```python
from build123d import *

# Parameters (mm, degrees)
V3_BOX_FOOTPRINT_100_X_45_MM_W                 = 100
V3_BOX_FOOTPRINT_100_X_45_MM_H                 = 45
V3_BOX_HEIGHT_35_MM_DEPTH                      = 35
V3_REAR_OPENING_96_X_31_MM_W                   = 96
V3_REAR_OPENING_96_X_31_MM_H                   = 31
V3_CAVITY_ALL_WALLS_2_MM_DEPTH                 = 43
V3_SQUARE_BEAMS_10_X_10_PITCH_95_MM_W          = 10
V3_SQUARE_BEAMS_10_X_10_PITCH_95_MM_H          = 10
V3_FORWARD_BEAM_LENGTH_65_MM_DEPTH             = 65
V3_LEFT_PCB_EAR_PROFILE_W                      = 10
V3_LEFT_PCB_EAR_PROFILE_H                      = 10
V3_LEFT_INWARD_EAR_5_MM_DEPTH                  = 5
V3_RIGHT_PCB_EAR_PROFILE_W                     = 10
V3_RIGHT_PCB_EAR_PROFILE_H                     = 10
V3_RIGHT_INWARD_EAR_5_MM_DEPTH                 = 5
V3_PCB_ROOF_PAIR_PITCH_85_MM_R                 = 1.7
V3_M3_ROOF_HOLES_DIAMETER_3_4_MM_DEPTH         = 2
V3_PCB_FORWARD_PAIR_ROW_SPACING_60_MM_R        = 1.7
V3_M3_PCB_EAR_HOLES_DEPTH                      = 10
V3_CHASSIS_TOP_HOLES_WIDTH_95_DEPTH_40_M_R     = 1.7
V3_M3_BEAM_TOP_BOTTOM_HOLES_DEPTH              = 10
V3_HANGING_PLATE_OFFSET_26_THICKNESS_2_5_W     = 110
V3_HANGING_PLATE_OFFSET_26_THICKNESS_2_5_H     = 2.5
V3_MOUNTING_PLATE_DOWNWARD_15_MM_WIDTH_1_DEPTH = 15
FOUR_HORIZONTAL_SLOTS_3_4_X_5_4_MM_DEPTH       = 2.5
CUT_EXTRUDE_1_DEPTH                            = 93.059763198
H_CROSSMEMBER_10_X_10_MM_AT_BEAM_MIDPOIN_W     = 10
H_CROSSMEMBER_10_X_10_MM_AT_BEAM_MIDPOIN_H     = 10
H_CROSSMEMBER_85_MM_DEPTH                      = 85
LONGITUDINAL_START                             = -2
BEAM_CAVITIES_6_MM_WIDE_PRESERVING_SCREW_W     = 6
BEAM_CAVITIES_6_MM_WIDE_PRESERVING_SCREW_H     = 6
BEAM_CAVITIES_6_MM_WIDE_PRESERVING_SCREW_H_2   = 27
BEAM_CAVITIES_6_MM_WIDE_PRESERVING_SCREW_H_3   = 9
LONGITUDINAL_BEAM_WALLS_2_MM_INNER_HEI_DEPTH   = 6
H_START                                        = -2
H_CROSSMEMBER_CAVITY_CONNECTS_BOTH_BEAM_W      = 89
H_CROSSMEMBER_CAVITY_CONNECTS_BOTH_BEAM_H      = 6
H_CROSSMEMBER_WALLS_2_MM_DEPTH                 = 6
CUT_EXTRUDE_4_DEPTH                            = 93.059763198
V6_EXTEND_10_X_10_HOLLOW_BEAMS_WITH_2_MM_W     = 10
V6_EXTEND_10_X_10_HOLLOW_BEAMS_WITH_2_MM_H     = 10
V6_EXTEND_10_X_10_HOLLOW_BEAMS_WITH_2_MM_W_2   = 6
V6_EXTEND_10_X_10_HOLLOW_BEAMS_WITH_2_MM_H_2   = 6
V6_HOLLOW_BEAM_EXTENSIONS_15_MM_DEPTH          = 15
V6_FOUR_FULL_DEPTH_PCB_PADS_CENTERS_X42_W      = 15
V6_FOUR_FULL_DEPTH_PCB_PADS_CENTERS_X42_H      = 10
V6_SOLID_SCREW_PADS_WITH_5_MM_INWARD_EAR_DEPTH = 10
V6_PCB_HOLES_85_X_60_MM_AND_RETAINED_CHA_R     = 1.7
V6_FOUR_PCB_M3_HOLES_THROUGH_REINFORCED_DEPTH  = 10


with BuildPart() as part:
    # V3 box footprint 100 x 45 mm → V3 box height 35 mm (new body)
    with BuildSketch(Plane.XY):
        with Locations((0, 22.5)):
            Rectangle(V3_BOX_FOOTPRINT_100_X_45_MM_W, V3_BOX_FOOTPRINT_100_X_45_MM_H)
    extrude(amount=V3_BOX_HEIGHT_35_MM_DEPTH)

    # V3 rear opening 96 x 31 mm → V3 cavity all walls 2 mm (cut)
    with BuildSketch(Plane(origin=(0, 45, 0), x_dir=(1, 0, 0), z_dir=(0, 1, 0))):
        with Locations((0, -17.5)):
            Rectangle(V3_REAR_OPENING_96_X_31_MM_W, V3_REAR_OPENING_96_X_31_MM_H)
    extrude(amount=-V3_CAVITY_ALL_WALLS_2_MM_DEPTH, mode=Mode.SUBTRACT)

    # V3 square beams 10 x 10 pitch 95 mm → V3 forward beam length 65 mm (add)
    with BuildSketch(Plane.XZ):
        with Locations((-47.5, 30)):
            Rectangle(V3_SQUARE_BEAMS_10_X_10_PITCH_95_MM_W, V3_SQUARE_BEAMS_10_X_10_PITCH_95_MM_H)
        with Locations((47.5, 30)):
            Rectangle(V3_SQUARE_BEAMS_10_X_10_PITCH_95_MM_W, V3_SQUARE_BEAMS_10_X_10_PITCH_95_MM_H)
    extrude(amount=V3_FORWARD_BEAM_LENGTH_65_MM_DEPTH)

    # V3 left PCB ear profile → V3 left inward ear 5 mm (add)
    with BuildSketch(Plane(origin=(-42.5, 0, 0), x_dir=(0, 0, -1), z_dir=(1, 0, 0))):
        with Locations((-30, -20)):
            Rectangle(V3_LEFT_PCB_EAR_PROFILE_W, V3_LEFT_PCB_EAR_PROFILE_H)
    extrude(amount=V3_LEFT_INWARD_EAR_5_MM_DEPTH)

    # V3 right PCB ear profile → V3 right inward ear 5 mm (add)
    with BuildSketch(Plane.ZY.offset(-42.5)):
        with Locations((30, -20)):
            Rectangle(V3_RIGHT_PCB_EAR_PROFILE_W, V3_RIGHT_PCB_EAR_PROFILE_H)
    extrude(amount=V3_RIGHT_INWARD_EAR_5_MM_DEPTH)

    # V3 PCB roof pair pitch 85 mm → V3 M3 roof holes diameter 3.4 mm (cut)
    with BuildSketch(Plane.XY.offset(35)):
        with Locations((-42.5, 40)):
            Circle(V3_PCB_ROOF_PAIR_PITCH_85_MM_R)
        with Locations((42.5, 40)):
            Circle(V3_PCB_ROOF_PAIR_PITCH_85_MM_R)
    extrude(amount=-V3_M3_ROOF_HOLES_DIAMETER_3_4_MM_DEPTH, mode=Mode.SUBTRACT)

    # V3 PCB forward pair row spacing 60 mm → V3 M3 PCB ear holes (cut)
    with BuildSketch(Plane.XY.offset(35)):
        with Locations((-42.5, -20)):
            Circle(V3_PCB_FORWARD_PAIR_ROW_SPACING_60_MM_R)
        with Locations((42.5, -20)):
            Circle(V3_PCB_FORWARD_PAIR_ROW_SPACING_60_MM_R)
    extrude(amount=-V3_M3_PCB_EAR_HOLES_DEPTH, mode=Mode.SUBTRACT)

    # V3 chassis top holes width 95 depth 40 mm → V3 M3 beam top bottom holes (cut)
    with BuildSketch(Plane.XY.offset(35)):
        with Locations((-47.5, -55)):
            Circle(V3_CHASSIS_TOP_HOLES_WIDTH_95_DEPTH_40_M_R)
        with Locations((-47.5, -15)):
            Circle(V3_CHASSIS_TOP_HOLES_WIDTH_95_DEPTH_40_M_R)
        with Locations((47.5, -55)):
            Circle(V3_CHASSIS_TOP_HOLES_WIDTH_95_DEPTH_40_M_R)
        with Locations((47.5, -15)):
            Circle(V3_CHASSIS_TOP_HOLES_WIDTH_95_DEPTH_40_M_R)
    extrude(amount=-V3_M3_BEAM_TOP_BOTTOM_HOLES_DEPTH, mode=Mode.SUBTRACT)

    # V3 hanging plate offset 26 thickness 2.5 mm → V3 mounting plate downward 15 mm width 110 (add)
    with BuildSketch(Plane(origin=(0, 0, 25), x_dir=(-1, 0, 0), z_dir=(0, 0, -1))):
        with Locations((0, -27.25)):
            Rectangle(V3_HANGING_PLATE_OFFSET_26_THICKNESS_2_5_W, V3_HANGING_PLATE_OFFSET_26_THICKNESS_2_5_H)
    extrude(amount=V3_MOUNTING_PLATE_DOWNWARD_15_MM_WIDTH_1_DEPTH)

    # V3 slots 6 mm below beam underside centers 20 and 47.5 → Four horizontal slots 3.4 x 5.4 mm (cut)
    with BuildSketch(Plane.XZ.offset(28.5)):
        with BuildLine():
            Line((-48.5, 20.7), (-46.5, 20.7))
            ThreePointArc((-46.5, 20.7), (-44.8, 19), (-46.5, 17.3))
            Line((-46.5, 17.3), (-48.5, 17.3))
            ThreePointArc((-48.5, 17.3), (-50.2, 19), (-48.5, 20.7))
        make_face()
        with BuildLine():
            Line((-21, 20.7), (-19, 20.7))
            ThreePointArc((-19, 20.7), (-17.3, 19), (-19, 17.3))
            Line((-19, 17.3), (-21, 17.3))
            ThreePointArc((-21, 17.3), (-22.7, 19), (-21, 20.7))
        make_face()
        with BuildLine():
            Line((19, 20.7), (21, 20.7))
            ThreePointArc((21, 20.7), (22.7, 19), (21, 17.3))
            Line((21, 17.3), (19, 17.3))
            ThreePointArc((19, 17.3), (17.3, 19), (19, 20.7))
        make_face()
        with BuildLine():
            Line((46.5, 20.7), (48.5, 20.7))
            ThreePointArc((48.5, 20.7), (50.2, 19), (48.5, 17.3))
            Line((48.5, 17.3), (46.5, 17.3))
            ThreePointArc((46.5, 17.3), (44.8, 19), (46.5, 20.7))
        make_face()
    extrude(amount=-FOUR_HORIZONTAL_SLOTS_3_4_X_5_4_MM_DEPTH, mode=Mode.SUBTRACT)

    # 草图2 → 切除-拉伸1 (cut, through all)
    with BuildSketch(Plane(origin=(0, 0, 0), x_dir=(-1, 0, 0), z_dir=(0, 0, -1))):
        with BuildLine():
            Line((-32.029979042, 6.459471041), (-21.029979042, 6.459471041))
            ThreePointArc((-21.029979042, 6.459471041), (-19.570508001, 5), (-21.029979042, 3.540528959))
            Line((-21.029979042, 3.540528959), (-32.029979042, 3.540528959))
            ThreePointArc((-32.029979042, 3.540528959), (-33.489450083, 5), (-32.029979042, 6.459471041))
        make_face()
        with BuildLine():
            Line((23.620107008, 6.558669056), (34.620107008, 6.558669056))
            ThreePointArc((34.620107008, 6.558669056), (36.178776063, 5), (34.620107008, 3.441330944))
            Line((34.620107008, 3.441330944), (23.620107008, 3.441330944))
            ThreePointArc((23.620107008, 3.441330944), (22.061437952, 5), (23.620107008, 6.558669056))
        make_face()
    extrude(amount=-CUT_EXTRUDE_1_DEPTH, mode=Mode.SUBTRACT)

    # H crossmember 10 x 10 mm at beam midpoint → H crossmember 85 mm (add)
    with BuildSketch(Plane(origin=(-42.5, 0, 0), x_dir=(0, 0, -1), z_dir=(1, 0, 0))):
        with Locations((-30, -32.5)):
            Rectangle(H_CROSSMEMBER_10_X_10_MM_AT_BEAM_MIDPOIN_W, H_CROSSMEMBER_10_X_10_MM_AT_BEAM_MIDPOIN_H)
    extrude(amount=H_CROSSMEMBER_85_MM_DEPTH)

    # Beam cavities 6 mm wide preserving screw collars → Longitudinal beam walls 2 mm - inner height 6 mm (cut)
    with BuildSketch(Plane.XY.offset(35).offset(LONGITUDINAL_START)):
        with Locations((-47.5, -62)):
            Rectangle(BEAM_CAVITIES_6_MM_WIDE_PRESERVING_SCREW_W, BEAM_CAVITIES_6_MM_WIDE_PRESERVING_SCREW_H)
        with Locations((-47.5, -37.5)):
            Rectangle(BEAM_CAVITIES_6_MM_WIDE_PRESERVING_SCREW_W, BEAM_CAVITIES_6_MM_WIDE_PRESERVING_SCREW_H_2)
        with Locations((-47.5, -6.5)):
            Rectangle(BEAM_CAVITIES_6_MM_WIDE_PRESERVING_SCREW_W, BEAM_CAVITIES_6_MM_WIDE_PRESERVING_SCREW_H_3)
        with Locations((47.5, -62)):
            Rectangle(BEAM_CAVITIES_6_MM_WIDE_PRESERVING_SCREW_W, BEAM_CAVITIES_6_MM_WIDE_PRESERVING_SCREW_H)
        with Locations((47.5, -37.5)):
            Rectangle(BEAM_CAVITIES_6_MM_WIDE_PRESERVING_SCREW_W, BEAM_CAVITIES_6_MM_WIDE_PRESERVING_SCREW_H_2)
        with Locations((47.5, -6.5)):
            Rectangle(BEAM_CAVITIES_6_MM_WIDE_PRESERVING_SCREW_W, BEAM_CAVITIES_6_MM_WIDE_PRESERVING_SCREW_H_3)
    extrude(amount=-LONGITUDINAL_BEAM_WALLS_2_MM_INNER_HEI_DEPTH, mode=Mode.SUBTRACT)

    # H crossmember cavity connects both beam cavities → H crossmember walls 2 mm (cut)
    with BuildSketch(Plane.XY.offset(35).offset(H_START)):
        with Locations((0, -32.5)):
            Rectangle(H_CROSSMEMBER_CAVITY_CONNECTS_BOTH_BEAM_W, H_CROSSMEMBER_CAVITY_CONNECTS_BOTH_BEAM_H)
    extrude(amount=-H_CROSSMEMBER_WALLS_2_MM_DEPTH, mode=Mode.SUBTRACT)

    # 草图8 → 切除-拉伸4 (cut, through all)
    with BuildSketch(Plane(origin=(0, 0, 0), x_dir=(-1, 0, 0), z_dir=(0, 0, -1))):
        with BuildLine():
            Line((-14.372732488, 6.733005515), (-3.372732488, 6.733005515))
            ThreePointArc((-3.372732488, 6.733005515), (-1.826093217, 5.186366244), (-3.372732488, 3.639726973))
            Line((-3.372732488, 3.639726973), (-14.372732488, 3.639726973))
            ThreePointArc((-14.372732488, 3.639726973), (-15.919371759, 5.186366244), (-14.372732488, 6.733005515))
        make_face()
        with BuildLine():
            Line((4.72350579, 6.686366244), (15.27649421, 6.686366244))
            ThreePointArc((15.27649421, 6.686366244), (16.77649421, 5.186366244), (15.27649421, 3.686366244))
            Line((15.27649421, 3.686366244), (4.72350579, 3.686366244))
            ThreePointArc((4.72350579, 3.686366244), (3.22350579, 5.186366244), (4.72350579, 6.686366244))
        make_face()
    extrude(amount=-CUT_EXTRUDE_4_DEPTH, mode=Mode.SUBTRACT)

    # V6 extend 10 x 10 hollow beams with 2 mm walls → V6 hollow beam extensions 15 mm (add)
    # profile 1 of 2: a face of its own
    with BuildSketch(Plane.XZ.offset(65)):
        with Locations((-47.5, 30)):
            Rectangle(V6_EXTEND_10_X_10_HOLLOW_BEAMS_WITH_2_MM_W, V6_EXTEND_10_X_10_HOLLOW_BEAMS_WITH_2_MM_H)
        with Locations((-47.5, 30)):
            Rectangle(V6_EXTEND_10_X_10_HOLLOW_BEAMS_WITH_2_MM_W_2, V6_EXTEND_10_X_10_HOLLOW_BEAMS_WITH_2_MM_H_2, mode=Mode.SUBTRACT)
    # profile 2 of 2: a face of its own
    with BuildSketch(Plane.XZ.offset(65)):
        with Locations((47.5, 30)):
            Rectangle(V6_EXTEND_10_X_10_HOLLOW_BEAMS_WITH_2_MM_W, V6_EXTEND_10_X_10_HOLLOW_BEAMS_WITH_2_MM_H)
        with Locations((47.5, 30)):
            Rectangle(V6_EXTEND_10_X_10_HOLLOW_BEAMS_WITH_2_MM_W_2, V6_EXTEND_10_X_10_HOLLOW_BEAMS_WITH_2_MM_H_2, mode=Mode.SUBTRACT)
    extrude(amount=V6_HOLLOW_BEAM_EXTENSIONS_15_MM_DEPTH)

    # V6 four full-depth PCB pads centers x42.5 y-70 and -10 → V6 solid screw pads with 5 mm inward ears (add)
    with BuildSketch(Plane.XY.offset(35)):
        with Locations((-45, -70)):
            Rectangle(V6_FOUR_FULL_DEPTH_PCB_PADS_CENTERS_X42_W, V6_FOUR_FULL_DEPTH_PCB_PADS_CENTERS_X42_H)
        with Locations((45, -70)):
            Rectangle(V6_FOUR_FULL_DEPTH_PCB_PADS_CENTERS_X42_W, V6_FOUR_FULL_DEPTH_PCB_PADS_CENTERS_X42_H)
        with Locations((-45, -10)):
            Rectangle(V6_FOUR_FULL_DEPTH_PCB_PADS_CENTERS_X42_W, V6_FOUR_FULL_DEPTH_PCB_PADS_CENTERS_X42_H)
        with Locations((45, -10)):
            Rectangle(V6_FOUR_FULL_DEPTH_PCB_PADS_CENTERS_X42_W, V6_FOUR_FULL_DEPTH_PCB_PADS_CENTERS_X42_H)
    extrude(amount=-V6_SOLID_SCREW_PADS_WITH_5_MM_INWARD_EAR_DEPTH)

    # V6 PCB holes 85 x 60 mm and retained chassis holes → V6 four PCB M3 holes through reinforced beam pads (cut)
    with BuildSketch(Plane.XY.offset(35)):
        with Locations((-42.5, -70)):
            Circle(V6_PCB_HOLES_85_X_60_MM_AND_RETAINED_CHA_R)
        with Locations((-42.5, -10)):
            Circle(V6_PCB_HOLES_85_X_60_MM_AND_RETAINED_CHA_R)
        with Locations((42.5, -70)):
            Circle(V6_PCB_HOLES_85_X_60_MM_AND_RETAINED_CHA_R)
        with Locations((42.5, -10)):
            Circle(V6_PCB_HOLES_85_X_60_MM_AND_RETAINED_CHA_R)
        with Locations((-47.5, -15)):
            Circle(V6_PCB_HOLES_85_X_60_MM_AND_RETAINED_CHA_R)
        with Locations((47.5, -15)):
            Circle(V6_PCB_HOLES_85_X_60_MM_AND_RETAINED_CHA_R)
    extrude(amount=-V6_FOUR_PCB_M3_HOLES_THROUGH_REINFORCED_DEPTH, mode=Mode.SUBTRACT)


solid = part.part
```
Verification items for the finished model (mm, model axes). A direction names the side the tool comes from. Coordinates: 2 decimals unless noted, no trailing zeros. Loops run counter-clockwise (first coordinate to the right, second up) from the corner with the lowest first, then second, coordinate; pieces in that order, holes last. Notation, with made-up numbers: (38, -5) - (84, -5) arc R25 cw to (84, 14) - close; hole circle Ø7 at (-3, -31). An arc over 180 degrees is marked (long way). Answer as a JSON object with one key per item and string values.
(1) Scan lines: line 1 along Y through (x, z) = (-47.5, 28.5); line 2 along X through (y, z) = (-15, 28); line 3 along X through (y, z) = (-70, 28.25). Record each from-to range of solid material in increasing order.
Response:
{"line 1": "y = -75 to -65, -59 to -56.7, -53.3 to -51, -24 to -16.7, -13.3 to -5, -2 to 2", "line 2": "x = -52.5 to -49.2, -45.8 to -37.5, 37.5 to 45.8, 49.2 to 52.5", "line 3": "x = -52.5 to -44.2, -40.8 to -37.5, 37.5 to 40.8, 44.2 to 52.5"}
(2) Cross-section at A-A, the plane y = -15. Record the boundary of the cut face in (x, z).
Response:
{"outline": "(-52.5, 25) - (-49.2, 25) - (-49.2, 35) - (-52.5, 35) - close; (-45.8, 25) - (-37.5, 25) - (-37.5, 35) - (-45.8, 35) - close; (37.5, 25) - (45.8, 25) - (45.8, 35) - (37.5, 35) - close; (49.2, 25) - (52.5, 25) - (52.5, 35) - (49.2, 35) - close"}
(3) Cross-section at B-B, the plane x = 39. Record the boundary of the cut face in (y, z), then the cut area to 4 significant figures.
Response:
{"outline": "(-75, 25) - (-65, 25) - (-65, 35) - (-75, 35) - close; (-37.5, 25) - (-28.5, 25) - (-28.5, 10) - (-26, 10) - (-26, 25) - (-27.5, 25) - (-27.5, 35) - (-37.5, 35) - close; (-25, 25) - (-5, 25) - (-5, 35) - (-25, 35) - close; (0, 0) - (45, 0) - (45, 2) - (2, 2) - (2, 33) - (45, 33) - (45, 35) - (0, 35) - close; hole (-35.5, 27) - (-29.5, 27) - (-29.5, 33) - (-35.5, 33) - close", "area": "643.5 mm²"}
(4) Go/stop test with flat-tipped pins: pin 1 Ø3 at (x, z) = (30, 9.5) entering from +Y; pin 2 Ø3 at (x, y) = (-42.5, -70) entering from +Z; pin 3 Ø1.5 at (x, z) = (-6.5, 4) entering from -Y; pin 4 Ø4 at (y, z) = (-77.5, 28.5) entering from -X. Record where each tip stops, or that it passes through.
Response:
{"pin 1": "stops at y = 2", "pin 2": "passes through", "pin 3": "stops at y = 0", "pin 4": "stops at x = -52.5"}
(5) Access from +Z, -Z, +X, -X, +Y, -Y to the whole of each face (thin tool, end or side, straight path). Record for faces 4 (the flat face through (-1, -27.5, 30)), 5 (the flat face through (-1, 24, 2)), 6 (the flat face through (47, -65, 30)), 7 (the flat face through (-40, -65, 30)), 8 (the flat face through (-40, -75, 30)).
Response:
{"face 4": "+Z", "face 5": "+Y", "face 6": "none", "face 7": "+Z, -Z", "face 8": "+Z, -Z, -Y"}
(6) Mould release check, pull along Z, two halves, no side actions. Record for faces 1 (the flat face through (-50.5, -77, 30)), 2 (the flat face through (42.5, -2, 30)), 3 (the flat face through (-1, 11, 35)): pulls with the +Z half, pulls with the -Z half, needs draft (parallel to the pull), parting line crosses it, or undercut.
Response:
{"face 1": "undercut", "face 2": "needs draft", "face 3": "pulls with the +Z half"}
(7) Cross-section at D-D, the plane z = 7. Record the boundary of the cut face in (x, y).
Response:
{"outline": "(-50, 0) - (50, 0) - (50, 45) - (48, 45) - (48, 2) - (-48, 2) - (-48, 45) - (-50, 45) - close"}
(8) Cross-section at C-C, the plane y = 13. Record the boundary of the cut face in (x, z).
Response:
{"outline": "(-50, 0) - (50, 0) - (50, 35) - (-50, 35) - close; hole (-48, 2) - (48, 2) - (48, 33) - (-48, 33) - close"}
